```python
from build123d import *

# Parameters (mm, degrees)
SKETCH_1_R          = 40
SKETCH_1_R_2        = 2.25
EXTRUDE_1_DEPTH     = 3
CUT_EXTRUDE_1_REACH = 58.648


with BuildPart() as part:
    # 草图1 → 凸台-拉伸1 (new body)
    with BuildSketch(Plane(origin=(0, 0, 0), x_dir=(1, 0, 0), z_dir=(0, 1, 0))):
        with Locations(Location((0, 0, 0), (0, 0, 270))):
            Circle(SKETCH_1_R)
        with Locations(Location((0, 0, 0), (0, 0, 270))):
            Circle(SKETCH_1_R_2, mode=Mode.SUBTRACT)
    extrude(amount=EXTRUDE_1_DEPTH)

    # 草图2 → 切除-拉伸1 (cut, up to next)
    with BuildSketch(Plane(origin=(0, 3, 0), x_dir=(1, 0, 0), z_dir=(0, 1, 0)), mode=Mode.PRIVATE) as cut_extrude_1_sk1:
        with BuildLine():
            Line((-37.5, 0), (-7.5, 0))
            ThreePointArc((-7.5, 0), (-5.303300859, 5.303300859), (0, 7.5))
            Line((0, 7.5), (0, 37.5))
            ThreePointArc((0, 37.5), (-26.516504294, 26.516504294), (-37.5, 0))
        make_face()
    cut_extrude_1_tool1 = extrude(cut_extrude_1_sk1.sketch, amount=-CUT_EXTRUDE_1_REACH, mode=Mode.PRIVATE) & part.part
    # 草图2 → 切除-拉伸1 (cut, up to next)
    with BuildSketch(Plane(origin=(0, 3, 0), x_dir=(1, 0, 0), z_dir=(0, 1, 0)), mode=Mode.PRIVATE) as cut_extrude_1_sk2:
        with BuildLine():
            Line((7.5, 0), (37.5, 0))
            ThreePointArc((37.5, 0), (26.516504294, -26.516504294), (0, -37.5))
            Line((0, -37.5), (0, -7.5))
            ThreePointArc((0, -7.5), (5.303300859, -5.303300859), (7.5, 0))
        make_face()
    cut_extrude_1_tool2 = extrude(cut_extrude_1_sk2.sketch, amount=-CUT_EXTRUDE_1_REACH, mode=Mode.PRIVATE) & part.part
    add(cut_extrude_1_tool1.solids().sort_by_distance((-16.446011, 3, -16.446011))[0], mode=Mode.SUBTRACT)
    add(cut_extrude_1_tool2.solids().sort_by_distance((16.446011, 3, 16.446011))[0], mode=Mode.SUBTRACT)


solid = part.part
```
Geometry: final body of the model. Coordinates: model frame, mm. A direction names the side the tool comes from. Give positions to 0.01 mm unless a question says otherwise; leave off trailing zeros. Write each loop counter-clockwise with the first axis right and the second up, starting at its lowest first coordinate (ties: lowest second). Pieces come first, ordered by that corner, then holes.
1. Section query C-C, the plane z = 19. Return loops of the section in (x, y).
2. Reachability of faces 5 (the flat face through (1, 0, -9)), 6 (the cylindrical face through (5.245, 1.521, 5.361)) from +Z, -Z, +X, -X, +Y, -Y: full face, straight path, thin tool, end or side. Return the list, or none.
3. Draft query along X for faces 1 (the flat face through (1, 3, -9)), 2 (the cylindrical face through (-5.361, 1.521, -5.245)), 3 (the flat face through (0, 2, -22)), 4 (the cylindrical face through (-39.05, 1.48, -8.67)). Return one class per face: released by +X, released by -X, zero draft, split by the parting line, or undercut.
4. Line query: probe 1 along X at (y, z) = (0.6, -1); probe 2 along X at (y, z) = (2.3, 0.5); probe 3 along Z at (x, y) = (-8.5, 2.05). Output: solid intervals per line, ascending.
5. Pin query (flat end, axial travel): P1, Ø1.5, axis at x = 25.5, y = 1.5, coming from the +Z side; P2, Ø0.9, axis at y = 2, z = 16, coming from the +X side; P3, Ø1.5, axis at x = -23, y = 1, coming from the -Z side; P4, Ø7, axis at x = 0, z = 0, coming from the -Y side. Return the tip coordinate at first contact, or that it passes through.
6. Section query A-A, the plane y = 1.9. Return loops of the section in (x, z).
7. Section query B-B, the plane x = -20. Return loops of the section in (y, z).
Computed:
1. outline: (-35.2, 0) - (0, 0) - (0, 3) - (-35.2, 3) - close; (32.33, 0) - (35.2, 0) - (35.2, 3) - (32.33, 3) - close
2. face 5: +Z, -Z, +X, -X, -Y
2. face 6: +Y, -Y
3. face 1: zero draft
3. face 2: undercut
3. face 3: undercut
3. face 4: split by the parting line
4. probe 1: x = -39.99 to -37.49, -7.43 to -2.02, 2.02 to 39.99
4. probe 2: x = -40 to -2.19, 2.19 to 7.48, 37.5 to 40
4. probe 3: z = -39.09 to -36.52, 0 to 39.09
5. P1: stops at z = 31.42
5. P2: stops at x = 36.85
5. P3: stops at z = -33.24
5. P4: stops at y = 0
6. outline: circle Ø80 at (0, 0); hole (-37.5, 0) arc R37.5 ccw to (0, -37.5) - (0, -7.5) arc R7.5 cw to (-7.5, 0) - close; hole circle Ø4.5 at (0, 0); hole (0, 7.5) arc R7.5 cw to (7.5, 0) - (37.5, 0) arc R37.5 ccw to (0, 37.5) - close
7. outline: (0, -34.64) - (3, -34.64) - (3, -31.72) - (0, -31.72) - close; (0, 0) - (3, 0) - (3, 34.64) - (0, 34.64) - close
